Autodesk Inventor part; units mm, degrees
ref_plane "YZ Plane" through (0, 0, 0) normal (1, 0, 0) x (0, 1, 0)
ref_plane "XZ Plane" through (0, 0, 0) normal (0, 1, 0) x (-1, 0, 0)
ref_plane "XY Plane" through (0, 0, 0) normal (0, 0, 1) x (1, 0, 0)
sketch "Sketch1" plane through (0, 0, 0) normal (0, 1, 0) x (-1, 0, 0)
  line L0 (-15, 15) -> (15, 15)
  line L1 (15, 15) -> (15, -15)
  line L2 (15, -15) -> (-15, -15)
  line L3 (-15, -15) -> (-15, 15)
  line L4 (-15, 15) -> (15, -15) construction
  line L5 (15, 15) -> (-15, -15) construction
  point P0 (0, 0)
  dimension "d0" = 30
  dimension "d1" = 30
extrude "Extrusion1" add sketch "Sketch1" along normal blind 5
sketch "Sketch2" plane through (0, 5, 0) normal (0, 1, 0) x (1, 0, 0)
  circle A0 centre (0, 0) radius 7
  dimension "d4" = 14
extrude "Extrusion2" add sketch "Sketch2" along normal blind 10
sketch "Sketch3" plane through (0, 5, 0) normal (0, 1, 0) x (1, 0, 0)
  line L0 (-15, -15) -> (15, -15)
  line L1 (0, -15) -> (0, 15) construction
  line L2 (15, 15) -> (-15, 15)
  line L3 (0, 0.1067) -> (-10, 0.1067) construction
  circle A0 centre (-10, 0.1067) radius 1.25
  point P0 (0, 0)
  point P1 (0, 0)
  dimension "d7" = 2.5
  dimension "d8" = 10
extrude "Extrusion3" add sketch "Sketch3" along normal blind 10.5
pattern_circular "Circular Pattern1" count 4 over 360 about axis through (0, 5, 0) along (0, 1, 0) of "Extrusion3"
sketch "Sketch4" plane through (0, 5, 0) normal (0, 1, 0) x (1, 0, 0)
  circle A0 centre (-10, 0.1067) radius 1.25
  circle A1 centre (-10, 0.1067) radius 2.5
  circle A2 centre (0.1067, 10) radius 1.25
  circle A3 centre (0.1067, 10) radius 2.5
  circle A4 centre (-0.1067, -10) radius 1.25
  circle A5 centre (-0.1067, -10) radius 2.5
  circle A6 centre (10, -0.1067) radius 1.25
  circle A7 centre (10, -0.1067) radius 2.5
  circle A8 centre (0, 0) radius 7
  circle A9 centre (0, 0) radius 8
  line L0 (15, -15) -> (-15, -15)
  line L1 (-15, -15) -> (-15, 15)
  line L2 (-15, 15) -> (15, 15)
  line L3 (15, 15) -> (15, -15)
  line L4 (15, -15) -> (-15, 15) construction
  line L5 (-15, -15) -> (15, 15) construction
  point P0 (7.8729, -1.4203)
  point P1 (1.2519, -7.9014)
  point P2 (-1.4203, -7.8729)
  point P3 (-7.9014, -1.2519)
  point P4 (-7.8729, 1.4203)
  point P5 (-1.2519, 7.9014)
  point P6 (1.4203, 7.8729)
  point P7 (7.9014, 1.2519)
  dimension "d14" = 5
  dimension "d15" = 5
  dimension "d16" = 5
  dimension "d17" = 5
  dimension "d18" = 16
extrude "Extrusion4" add sketch "Sketch4" along normal up to surface (10.5 mm away) contours L0 L1 L2 L3
fillet "Fillet1" radius 1 8 edges at (-1.2519, 10.25, -7.9014) (-7.8729, 10.25, -1.4203) (-7.9014, 10.25, 1.2519) (-1.4203, 10.25, 7.8729) (1.2519, 10.25, 7.9014) (7.8729, 10.25, 1.4203) (7.9014, 10.25, -1.2519) (1.4203, 10.25, -7.8729)
fillet "Fillet2" radius 2 4 edges at (15, 7.75, 15) (15, 7.75, -15) (-15, 7.75, 15) (-15, 7.75, -15)
equation "\"d1\" = d0"
equation "\"d15\" = d14"
equation "\"d16\" = d14"
equation "\"d17\" = d14"
properties part number "PDMS stretcher mould A (x4) V2"
The model under review builds one solid part; all positions refer to its coordinate system, in mm. A direction names the side the tool comes from. Round coordinates to 2 decimals unless told otherwise and drop trailing zeros. Loops run counter-clockwise (first coordinate to the right, second up) from the corner with the lowest first, then second, coordinate; pieces in that order, holes last. Notation, with made-up numbers: (40, 7) -> (73, 7) arc R33 ccw to (73, 46) -> close; hole circle Ø7 at (-27, -5.5). An arc over 180 degrees is marked (long way). Answer as a JSON object with one key per item and string values. Group by question number.
1) For line 1 (Z direction, x = -10, y = 10.75); line 2 (Z direction, x = 10, y = 8.75); line 3 (X direction, y = 12, z = -11), list the stretches that pass through material, from the lowest coordinate up. Write a range as [from, to].
2) We need section C-C on y = 11.75. Give the number of separate pieces and of enclosed holes in the cut face, then the cut area to 3 significant figures.
3) For pin 1 Ø3 at (x, z) = (-2, 2.5) entering from +Y; pin 2 Ø6 at (x, z) = (0.11, -10) entering from -Y, all flat-tipped, find the tip position at first contact; note any pin that passes through.
4) For faces 1 (the face through (5.683, 10.176, -5.63)), 2 (the face through (0, 0, 0)), list the 3-axis set-ups (+Z, -Z, +X, -X, +Y, -Y) from which the entire face can be reached by the end or side of a thin tool; tool diameter is ignored.
5) We need section B-B on z = -6. Write out the cut boundary in (x, y), then the cut area to 3 significant figures.
6) We need section A-A on x = 5.5. Write out the cut boundary in (y, z).
7) Mouldability with a two-part tool opening along Z and no side actions: class faces 3 (the face through (0, 8, -15)), 4 (the face through (3, 5, 7)), 5 (the face through (0, 15.5, 10)) as released by +Z, released by -Z, zero draft, split by the parting line, or undercut.
Result set:
{
 "1": {"line 1": "[-15, -2.61], [-1.36, 1.14], [2.39, 15]", "line 2": "[-15, -2.39], [-1.14, 1.36], [2.61, 15]", "line 3": "[-15, -2.18], [-0.64, 0.86], [2.4, 15]"},
 "2": {"separate pieces": "6", "enclosed holes": "1", "area": "791 mm²"},
 "3": {"pin 1": "y = 15", "pin 2": "y = 0"},
 "4": {"face 1": "+Y", "face 2": "+Z, -Z, +X, -X, -Y"},
 "5": {"outline": "(-15, 0) -> (15, 0) -> (15, 15.5) -> (5.29, 15.5) -> (5.29, 5) -> (3.61, 5) -> (3.61, 15) -> (-3.61, 15) -> (-3.61, 5) -> (-5.29, 5) -> (-5.29, 15.5) -> (-15, 15.5) -> close", "area": "426 mm²"},
 "6": {"outline": "(0, -15) -> (15.5, -15) -> (15.5, -5.81) -> (5, -5.81) -> (5, -4.33) -> (15, -4.33) -> (15, 4.33) -> (5, 4.33) -> (5, 5.81) -> (15.5, 5.81) -> (15.5, 15) -> (0, 15) -> close"},
 "7": {"face 3": "released by -Z", "face 4": "undercut", "face 5": "zero draft"}
}
